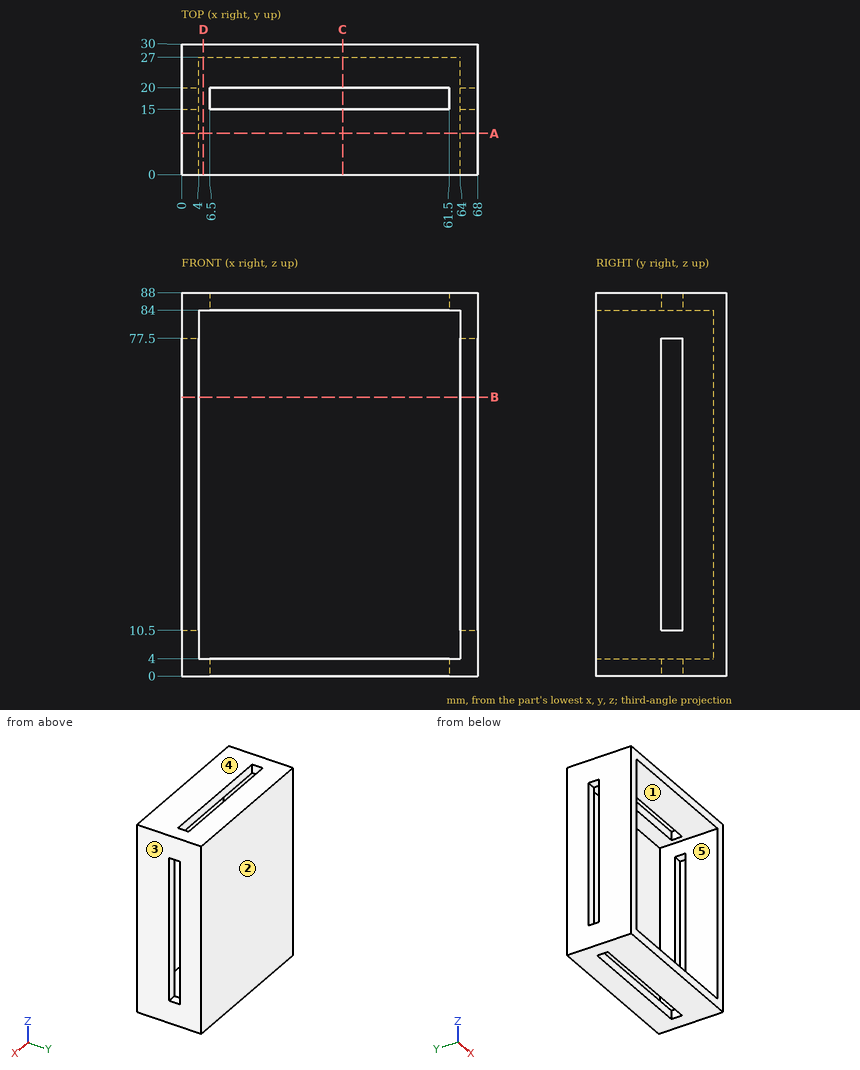
Source: three-view drawing plus pictorial views. Frame: mm from the lowest corner of the part. A direction names the side the tool comes from. Give positions to 0.01 mm unless a question says otherwise; leave off trailing zeros. Order: outer loops, then holes, each group sorted by start corner. A loop starts at its lowest first (then second) coordinate and runs counter-clockwise, first axis right, second up. Notation, with made-up numbers: (72.25, -39) - (85.25, -39) arc R11 ccw to (85.25, -22) - close; hole circle Ø11 at (-19, 87). An arc over 180 degrees is marked (long way). Answer as a JSON object with one key per item and string values. Group by question number.
Q1. Cut plane D-D, the plane x = 5. Output: boundary loops of the cut face in (y, z).
Q2. Line query: probe 1 along X at (y, z) = (7.25, 64); probe 2 along Z at (x, y) = (23, 9.5); probe 3 along Y at (x, z) = (37, 67.5). Output: solid intervals per line, ascending.
Q3. Mould query, pull axis X, two halves, no side actions, for the marked faces 3, 4 and 5. Classes: pulls with the +X half, pulls with the -X half, needs draft (parallel to the pull), parting line crosses it, or undercut.
Q4. Cut plane A-A, the plane y = 9.5. Output: boundary loops of the cut face in (x, z), then the cut area to 3 significant figures.
Q5. Cut plane C-C, the plane x = 37. Output: boundary loops of the cut face in (y, z).
Q6. Set-up query: the marked faces 1 and 2. Return all of +Z, -Z, +X, -X, +Y, -Y with unobstructed straight access to the full face (end or side cutting, diameter ignored); none if empty.
Q7. Cut plane B-B, the plane z = 64. Output: boundary loops of the cut face in (x, y), then the cut area to 3 significant figures.
Q8. First-contact query: pin 1 Ø2 at (x, z) = (26, 86) entering from -Y; pin 2 Ø1.5 at (y, z) = (16, 74.5) entering from +X; pin 3 Ø1 at (x, z) = (23, 65) entering from -Y. Flat tips, straight axial feed; report the tip coordinate or a pass-through.
Results:
{
 "1": {"outline": "(0, 0) - (30, 0) - (30, 88) - (0, 88) - (0, 84) - (27, 84) - (27, 4) - (0, 4) - close"},
 "2": {"probe 1": "0 to 4, 64 to 68", "probe 2": "0 to 4, 84 to 88", "probe 3": "27 to 30"},
 "3": {"face 3": "pulls with the +X half", "face 4": "needs draft", "face 5": "undercut"},
 "4": {"outline": "(0, 0) - (68, 0) - (68, 88) - (0, 88) - close; hole (4, 4) - (64, 4) - (64, 84) - (4, 84) - close", "area": "1,180 mm^2"},
 "5": {"outline": "(0, 0) - (15, 0) - (15, 4) - (0, 4) - close; (0, 84) - (15, 84) - (15, 88) - (0, 88) - close; (20, 0) - (30, 0) - (30, 88) - (20, 88) - (20, 84) - (27, 84) - (27, 4) - (20, 4) - close"},
 "6": {"face 1": "-Y", "face 2": "+Z, -Z, +X, -X, +Y"},
 "7": {"outline": "(0, 0) - (4, 0) - (4, 15) - (0, 15) - close; (0, 20) - (4, 20) - (4, 27) - (64, 27) - (64, 20) - (68, 20) - (68, 30) - (0, 30) - close; (64, 0) - (68, 0) - (68, 15) - (64, 15) - close", "area": "380 mm^2"},
 "8": {"pin 1": "y = 0", "pin 2": "through", "pin 3": "y = 27"}
}
